Geometry check sheet. Reference: the model listing, model coordinates, mm. A direction names the side the tool comes from. Round coordinates to 2 decimals unless told otherwise and drop trailing zeros. Write each loop counter-clockwise with the first axis right and the second up, starting at its lowest first coordinate (ties: lowest second). Pieces come first, ordered by that corner, then holes. Notation, with made-up numbers: M -29,8.5 L -20,8.5 A19 cw -20,19.5 Z; hole C 52,42 d4. An arc over 180 degrees is marked long. One line per item, written item: value. Start each with the question number.
1. Section check D-D (z = -6). Record the boundary of the cut face in (x, y).
2. Depth check by flat-ended pin: P1, Ø1.5, axis at y = 2.5, z = -3, coming from the +X side; P2, Ø4, axis at x = 3.5, z = 7.5, coming from the +Y side. Enter the tip coordinate at first touch or a pass-through.
3. Section check C-C (x = 15). Record the boundary of the cut face in (y, z).
4. Section check A-A (y = 6). Record the boundary of the cut face in (x, z), and give its area (3 significant figures).
5. Access from +Z, -Z, +X, -X, +Y, -Y to the whole of each face (thin tool, end or side, straight path). Record for faces 5 (the cylindrical face through (6.285, 2.711, -8.449)), 6 (the flat face through (5.7, 0, 0.2)).
6. Scan lines: probe 1 along Z at (x, y) = (3, 2.3) (3 decimals); probe 2 along Z at (x, y) = (16.25, 4.25); probe 3 along Y at (x, z) = (1.5, 1.5). Record each from-to range of solid material in increasing order. Write a range as [from, to].
7. Release check for a two-part mould opening along X. For faces 1 (the cylindrical face through (19.51, 11.24, -11.83)), 2 (the flat face through (20, 5, 12)), 3 (the cylindrical face through (2.67, 2.46, -13.34)), 4 (the flat face through (3, 5, 0)) record: pulls with the +X half, pulls with the -X half, needs draft (parallel to the pull), parting line crosses it, or undercut.
8. Section check B-B (x = 3). Record the boundary of the cut face in (y, z) (3 decimals), and give its area (3 significant figures).
from build123d import *

# Parameters (mm, degrees)
BOSS_EXTRUDE1_DEPTH = 15
SKETCH2_R           = 1.5
CUT_EXTRUDE1_DEPTH  = 30


with BuildPart() as part:
    # Sketch1 → Boss-Extrude1 (new, symmetric)
    with BuildSketch(Plane.XY):
        with BuildLine():
            Line((0, 0), (0, 4))
            ThreePointArc((0, 4), (0.292893219, 4.707106781), (1, 5))
            Line((1, 5), (5.763932023, 5))
            ThreePointArc((5.763932023, 5), (5.993684943, 5.026751011), (6.211145618, 5.105572809))
            Line((6.211145618, 5.105572809), (18.552786405, 11.276393202))
            ThreePointArc((18.552786405, 11.276393202), (19.525731112, 11.23261682), (20, 10.381966011))
            Line((20, 10.381966011), (20, 0))
            Line((20, 0), (0, 0))
        make_face()
    extrude(amount=BOSS_EXTRUDE1_DEPTH, both=True)

    # Sketch2 → Cut-Extrude1 (cut)
    with BuildSketch(Plane.XZ):
        with Locations((3, 11.875)):
            Circle(SKETCH2_R)
        with Locations((3, -11.875)):
            Circle(SKETCH2_R)
        with BuildLine():
            Line((20, -8.75), (20, 8.75))
            Line((20, 8.75), (7, 8.75))
            ThreePointArc((7, 8.75), (6.292893219, 8.457106781), (6, 7.75))
            Line((6, 7.75), (6, -7.75))
            ThreePointArc((6, -7.75), (6.292893219, -8.457106781), (7, -8.75))
            Line((7, -8.75), (20, -8.75))
        make_face()
    extrude(amount=-CUT_EXTRUDE1_DEPTH, mode=Mode.SUBTRACT)


solid = part.part
Result sheet:
1. outline: M 0,0 L 6,0 L 6,5.03 A1 cw 5.76,5 L 1,5 A1 ccw 0,4 Z
2. P1: stops at x = 6
2. P2: stops at y = 5
3. outline: M 0,-15 L 9.5,-15 L 9.5,-8.75 L 0,-8.75 Z; M 0,8.75 L 9.5,8.75 L 9.5,15 L 0,15 Z
4. outline: M 8,-15 L 20,-15 L 20,-8.75 L 8,-8.75 Z; M 8,8.75 L 20,8.75 L 20,15 L 8,15 Z
4. area: 150 mm2
5. face 5: +X, +Y, -Y
5. face 6: +Z, -Z, +X, -X, -Y
6. probe 1: z = [-15, -13.375], [-10.375, 10.375], [13.375, 15]
6. probe 2: z = [-15, -8.75], [8.75, 15]
6. probe 3: y = [0, 5]
7. face 1: parting line crosses it
7. face 2: pulls with the +X half
7. face 3: undercut
7. face 4: needs draft
8. outline: M 0,-15 L 5,-15 L 5,-13.375 L 0,-13.375 Z; M 0,-10.375 L 5,-10.375 L 5,10.375 L 0,10.375 Z; M 0,13.375 L 5,13.375 L 5,15 L 0,15 Z
8. area: 120 mm2
